from build123d import *

# Parameters (mm, degrees)
F2_R      = 68
F3_DEPTH  = 500
F1_FACE_R = 68.2
F4_DEPTH  = 200


with BuildPart() as f1:
    # F0 (on Front) → F1 (revolve)
    with BuildSketch(Plane.XZ):
        Polygon((-249.4, 169), (-114, 169), (-112, 168), (-112, 156), (0, 156), (0, 371), (-68.2, 371), (-68.2, 250), (-74.4, 250), (-74.4, 371), (-249.4, 371), align=None)
    revolve(axis=Axis((0, 0, 263.5), (0, 0, -1)))

    # F2 (on Front) → F3 (join)
    with BuildSketch(Plane.XZ):
        with Locations((-181.4, 270)):
            Circle(F2_R)
    extrude(amount=F3_DEPTH)

    # F1_face (on face) → F4 (join)
    with BuildSketch(Plane.XY.offset(371)):
        Circle(F1_FACE_R)
    extrude(amount=F4_DEPTH)


solid = f1.part
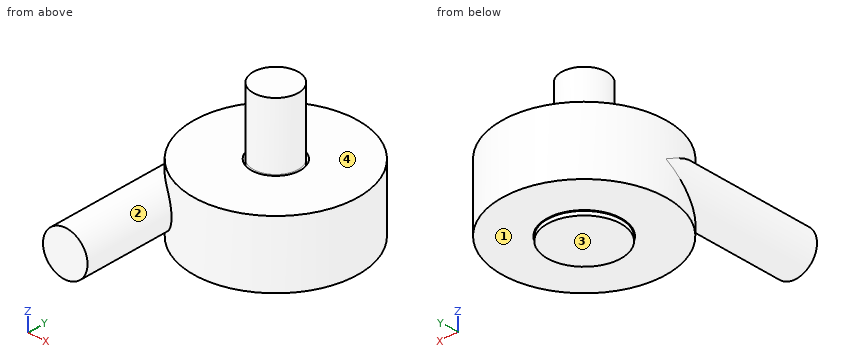
The listing builds one solid part. Answer for the finished solid, in the listing's coordinates (mm). Face numbers are marked on the shaded views. A direction names the side the tool comes from. Coordinates: 2 decimals unless noted, no trailing zeros. Write each loop counter-clockwise with the first axis right and the second up, starting at its lowest first coordinate (ties: lowest second). Pieces come first, ordered by that corner, then holes. Notation, with made-up numbers: M -19.75,62.5 L 38.25,62.5 A16 ccw 38.25,88.5 Z; hole C 55,15 d1. An arc over 180 degrees is marked long. Write each question's results on one line, items separated by ' | '.
Item 1: The part is cut by section A-A on z = 361. Determine the outline of the cut face in (x, y), and give its area (3 significant figures).
Answer below:
outline: C 0,0 d498.8; C 0,0 d136.4; hole C 0,0 d148.8 | area: 193,000 mm2
Item 2: The part is cut by section B-B on x = 0. Determine the outline of the cut face in (y, z), and give its area (3 significant figures).
Answer below:
outline: M -249.4,169 L -114,169 L -112,168 L -112,156 L 112,156 L 112,168 L 114,169 L 249.4,169 L 249.4,371 L 74.4,371 L 74.4,250 L 68.2,250 L 68.2,571 L -68.2,571 L -68.2,250 L -74.4,250 L -74.4,371 L -249.4,371 Z | area: 129,000 mm2
Item 3: The part is cut by section C-C on y = -239. Determine the outline of the cut face in (x, z), and give its area (3 significant figures).
Answer below:
outline: C -181.4,270 d136; M -71.27,169 L 71.27,169 L 71.27,371 L -71.27,371 Z | area: 43,300 mm2
Item 4: Given P1, Ø8, axis at x = -46, z = 490, coming from the -Y side; P2, Ø10, axis at y = -161.5, z = 249.5, coming from the +X side; P3, Ø4, axis at y = -155.5, z = 220.5, coming from the +X side, each flat-ended and moving along its own axis, determine where each tip first touches the part or whether it passes through.
Answer below:
P1: y = -53.73 | P2: x = 194.19 | P3: x = 196.57
Item 5: The part is cut by section D-D on z = 444.5. Determine the outline of the cut face in (x, y).
Answer below:
outline: C 0,0 d136.4
Item 6: Consider probe 1 along Y at (x, z) = (0, 275.5); probe 2 along Y at (x, z) = (13, 312); probe 3 along Z at (x, y) = (-119.5, -174.5). Determine where each line is inside the solid, lowest interval first. Write a range as [from, to].
Answer below:
probe 1: [-249.4, -74.4], [-68.2, 68.2], [74.4, 249.4] | probe 2: [-249.06, -73.26], [-66.95, 66.95], [73.26, 249.06] | probe 3: [169, 371]
Item 7: Which of the six approach directions +Z, -Z, +X, -X, +Y, -Y give full straight-line access (tool end or side, diameter ignored) to the marked faces 1, 2, 3 and 4?
Answer below:
face 1: -Z | face 2: -Y | face 3: -Z, +X, -X, +Y, -Y | face 4: +Z
